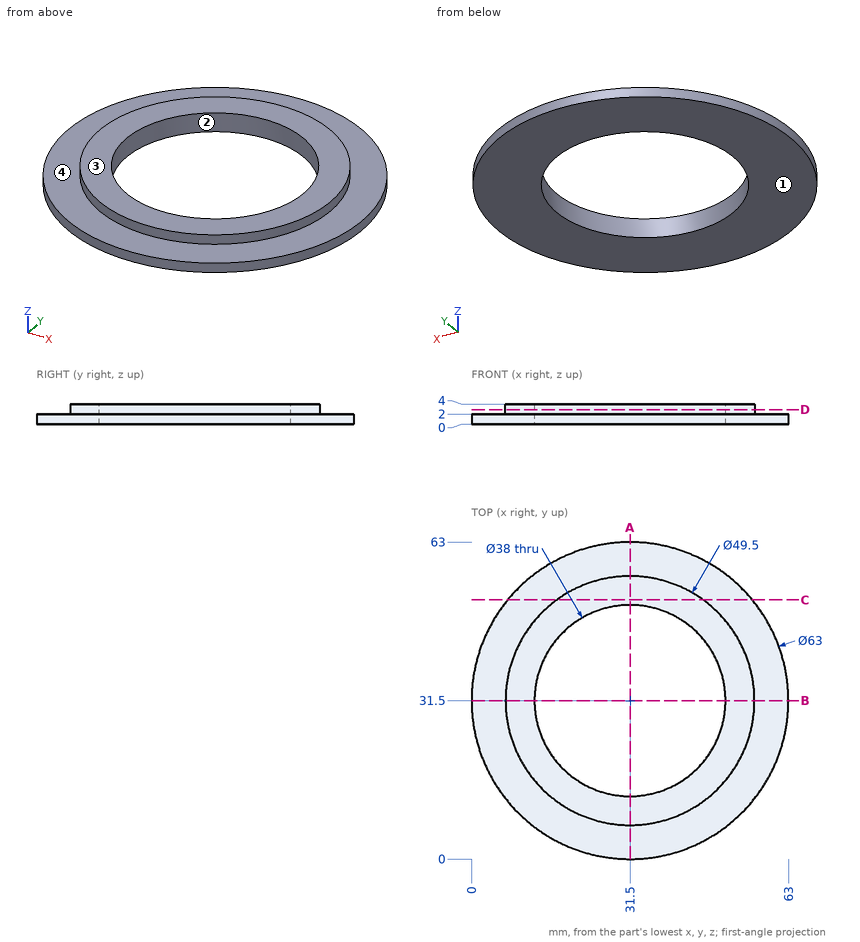
Geometry: see drawing. Coordinates: mm, zero at the bounding-box minimum. A direction names the side the tool comes from. Give positions to 0.01 mm unless a question says otherwise; leave off trailing zeros. Order: outer loops, then holes, each group sorted by start corner. A loop starts at its lowest first (then second) coordinate and runs counter-clockwise, first axis right, second up. Notation, with made-up numbers: (8, 46) -> (56, 46) arc R35 ccw to (56, 83) -> close; hole circle Ø7 at (21.25, -26.75). An arc over 180 degrees is marked (long way). Write each question's results on one line, items separated by ' | '.
1) Line query: line 1 along Y through (x, z) = (31.5, 1); line 2 along Y through (x, z) = (31.5, 2.05). Output: solid intervals per line, ascending.
Geometry says:
line 1: y = 0 to 12.5, 50.5 to 63 | line 2: y = 6.75 to 12.5, 50.5 to 56.25
2) Cut plane A-A (x = 31.5). Output: boundary loops of the cut face in (y, z), and give its area (3 significant figures).
Geometry says:
outline: (0, 0) -> (12.5, 0) -> (12.5, 4) -> (6.75, 4) -> (6.75, 2) -> (0, 2) -> close; (50.5, 0) -> (63, 0) -> (63, 2) -> (56.25, 2) -> (56.25, 4) -> (50.5, 4) -> close | area: 73.0 mm²
3) Set-up query: the marked faces 3 and 4. Return all of +Z, -Z, +X, -X, +Y, -Y with unobstructed straight access to the full face (end or side cutting, diameter ignored); none if empty.
Geometry says:
face 3: +Z, +X, -X, +Y, -Y | face 4: +Z
4) Draft query along Y for the marked faces 1 and 2. Return one class per face: released by +Y, released by -Y, zero draft, split by the parting line, or undercut.
Geometry says:
face 1: zero draft | face 2: undercut
5) Cut plane D-D (z = 2.9). Output: boundary loops of the cut face in (x, y), and give its area (3 significant figures).
Geometry says:
outline: circle Ø49.5 at (31.5, 31.5); hole circle Ø38 at (31.5, 31.5) | area: 790 mm²
6) First-contact query: pin 1 Ø1.5 at (x, z) = (17.5, 3) entering from +Y. Flat tip, straight axial feed; report the tip coordinate or a pass-through.
Geometry says:
pin 1: stops at y = 52.4
7) Cut plane C-C (y = 51.5). Output: boundary loops of the cut face in (x, z).
Geometry says:
outline: (7.16, 0) -> (55.84, 0) -> (55.84, 2) -> (46.08, 2) -> (46.08, 4) -> (16.92, 4) -> (16.92, 2) -> (7.16, 2) -> close
